Can you work these out from the model? Positions are in its coordinate system, mm. Face numbers are marked on the shaded views. Coordinates: 2 decimals unless noted, no trailing zeros. Order: outer loops, then holes, each group sorted by start corner. A loop starts at its lowest first (then second) coordinate and runs counter-clockwise, first axis right, second up. Notation, with made-up numbers: (53, 32.25) -> (58, 32.25) arc R21 cw to (58, 41.25) -> close; hole circle Ø1 at (-8, 33.5). An arc over 180 degrees is marked (long way). Answer in a Markdown table with one row per item.
```python
from build123d import *

# Parameters (mm, degrees)
F0_W     = 145
F0_H     = 30
F1_DEPTH = 3
F2_W     = 10
F2_H     = 3
F3_DEPTH = 25
F4_DEPTH = 5
F5_DEPTH = 5
F6_W     = 3
F6_H     = 12
F7_DEPTH = 25
F8_R     = 8
F9_DEPTH = 25


with BuildPart() as f1:
    # F0 (on Front) → F1 (new body)
    with BuildSketch(Plane.XZ):
        Rectangle(F0_W, F0_H)
    extrude(amount=F1_DEPTH)

    # F2 (on face) → F3 (cut)
    with BuildSketch(Plane.XZ.offset(3)):
        with Locations((-70, -13.5)):
            Rectangle(F2_W, F2_H)
        with Locations((-70, 13.5)):
            Rectangle(F2_W, F2_H)
        with Locations((-50, -13.5)):
            Rectangle(F2_W, F2_H)
        with Locations((-50, 13.5)):
            Rectangle(F2_W, F2_H)
        with Locations((-30, -13.5)):
            Rectangle(F2_W, F2_H)
        with Locations((-30, 13.5)):
            Rectangle(F2_W, F2_H)
        with Locations((-10, -13.5)):
            Rectangle(F2_W, F2_H)
        with Locations((-10, 13.5)):
            Rectangle(F2_W, F2_H)
        with Locations((10, -13.5)):
            Rectangle(F2_W, F2_H)
        with Locations((10, 13.5)):
            Rectangle(F2_W, F2_H)
        with Locations((30, -13.5)):
            Rectangle(F2_W, F2_H)
        with Locations((30, 13.5)):
            Rectangle(F2_W, F2_H)
        with Locations((50, -13.5)):
            Rectangle(F2_W, F2_H)
        with Locations((50, 13.5)):
            Rectangle(F2_W, F2_H)
        with Locations((70, -13.5)):
            Rectangle(F2_W, F2_H)
        with Locations((70, 13.5)):
            Rectangle(F2_W, F2_H)
    extrude(amount=-F3_DEPTH, mode=Mode.SUBTRACT)

    # F4 (add): faces of the model
    f4_faces = [f1.faces().sort_by_distance(p)[0] for p in [
        (72.5, -1.5, 0),
        (-72.5, -1.5, 0),
    ]]
    extrude(f4_faces, amount=F4_DEPTH, dir=(1, 0, 0))

    # F5 (add): a face of the model
    f5_faces = [f1.faces().sort_by_distance(p)[0] for p in [
        (-72.5, -1.5, 0),
    ]]
    extrude(f5_faces, amount=F5_DEPTH)

    # F6 (on face) → F7 (cut)
    with BuildSketch(Plane(origin=(0, 0, 0), x_dir=(-1, 0, 0), z_dir=(0, 1, 0))):
        with Locations((-74, -6)):
            Rectangle(F6_W, F6_H)
        with Locations((74, -6)):
            Rectangle(F6_W, F6_H)
    extrude(amount=-F7_DEPTH, mode=Mode.SUBTRACT)

    # F8 (on face) → F9 (cut)
    with BuildSketch(Plane.XZ.offset(3)):
        with Locations((-12.8, 2)):
            Circle(F8_R)
        with Locations((12.8, 2)):
            Circle(F8_R)
    extrude(amount=-F9_DEPTH, mode=Mode.SUBTRACT)


solid = f1.part
```
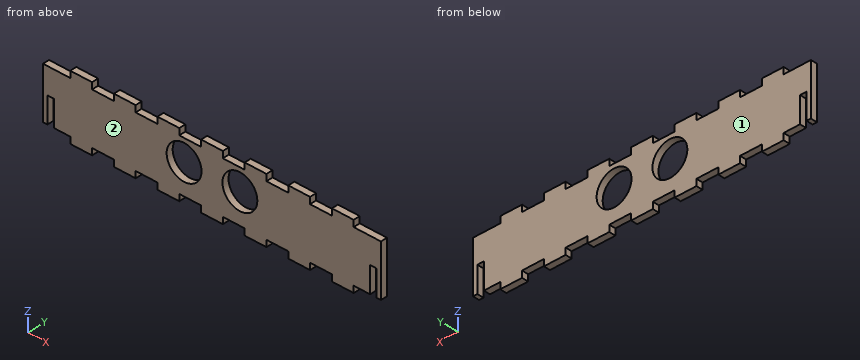
(1) I need wall thicknesses on line 1 (Z direction, x = 12.8, y = -0.9); line 2 (X direction, y = -0.2, z = -9.5); line 3 (X direction, y = -1.15, z = 0.5). Which ranges of each line are inside material? Lowest first, please. Write a range as [from, to].
Response values:
| item | result |
|---|---|
| line 1 | [-12, -6], [10, 12] |
| line 2 | [-77.5, -75.5], [-72.5, 72.5], [75.5, 77.5] |
| line 3 | [-77.5, -20.66], [-4.94, 4.94], [20.66, 77.5] |
(2) Suppose I cut it at C-C (y = -0.7). Count the separate pieces of the cut face and the enclosed holes in it, and give its area (3 significant figures).
Response values:
| item | result |
|---|---|
| separate pieces | 1 |
| enclosed holes | 2 |
| area | 3,670 mm2 |
(3) Will these pins go through, and if not, where does the flat tip stop? pin 1 Ø0.9 at (x, y) = (51, -1) entering from -Z; pin 2 Ø0.9 at (y, z) = (-2, 13) entering from -X; pin 3 Ø1.5 at (y, z) = (-1.5, 13) entering from +X; pin 4 Ø9.5 at (x, z) = (-12.8, 2) entering from -Y.
Response values:
| item | result |
|---|---|
| pin 1 | z = -12 |
| pin 2 | x = -65 |
| pin 3 | x = 65 |
| pin 4 | through |
(4) Suppose I cut it at A-A (z = 2). Please give me the cut outline in (x, y), and give its area (3 significant figures).
Response values:
| item | result |
|---|---|
| outline | (-77.5, -3) -> (-20.8, -3) -> (-20.8, 0) -> (-77.5, 0) -> close; (-4.8, -3) -> (4.8, -3) -> (4.8, 0) -> (-4.8, 0) -> close; (20.8, -3) -> (77.5, -3) -> (77.5, 0) -> (20.8, 0) -> close |
| area | 369 mm2 |
(5) Suppose I cut it at D-D (z = -9.75). Please give me the cut outline in (x, y), and give its area (3 significant figures).
Response values:
| item | result |
|---|---|
| outline | (-77.5, -3) -> (-75.5, -3) -> (-75.5, 0) -> (-77.5, 0) -> close; (-72.5, -3) -> (72.5, -3) -> (72.5, 0) -> (-72.5, 0) -> close; (75.5, -3) -> (77.5, -3) -> (77.5, 0) -> (75.5, 0) -> close |
| area | 447 mm2 |
(6) Suppose I cut it at B-B (x = -12.8). Please give me the cut outline in (y, z).
Response values:
| item | result |
|---|---|
| outline | (-3, -12) -> (0, -12) -> (0, -6) -> (-3, -6) -> close; (-3, 10) -> (0, 10) -> (0, 12) -> (-3, 12) -> close |
(7) We'd pull the mould along Y, two halves only. Please class the marked faces 1 and 2: +Y half, -Y half, draft (parallel to the pull), parting line (faces both ways), or undercut.
Response values:
| item | result |
|---|---|
| face 1 | +Y half |
| face 2 | -Y half |
